Source: CAD feature listing. Evaluate the final solid. Frame: model axes, mm. A direction names the side the tool comes from. Coordinates: 2 decimals unless noted, no trailing zeros. Order: outer loops, then holes, each group sorted by start corner. A loop starts at its lowest first (then second) coordinate and runs counter-clockwise, first axis right, second up.
```python
from build123d import *

# Parameters (mm, degrees)
SKETCH1_R                     = 31.5
EXTRUDE1_DEPTH                = 4
EXTRUDE_THIN1_DEPTH           = 13
CIRPATTERN7_COUNT             = 6
SKETCH3_R                     = 7
EXTRUDE2_DEPTH                = 6
M11_0_11_DIAMETER_HOLE1_D     = 11
M11_0_11_DIAMETER_HOLE1_DEPTH = 10
M11_0_11_DIAMETER_HOLE1_TIP   = 3.304733405


with BuildPart() as part:
    # Sketch1 → Extrude1 (new body)
    with BuildSketch(Plane.XY):
        Circle(SKETCH1_R)
    extrude(amount=EXTRUDE1_DEPTH)

    # Sketch2 → Extrude-Thin1 (add)
    with BuildSketch(Plane.XY.offset(4)):
        with BuildLine():
            ThreePointArc((10, -1), (20.741698661, 1.955169442), (28.460203071, 9.988960964))
            Line((28.460203071, 9.988960964), (26.702088493, 10.942393254))
            ThreePointArc((26.702088493, 10.942393254), (19.718679741, 3.673724733), (10, 1))
            Line((10, 1), (10, -1))
        make_face()
    extrude_thin1 = extrude(amount=EXTRUDE_THIN1_DEPTH)

    # CirPattern7: Extrude-Thin1 ×6 about axis
    cirpattern7_axis = Axis((0, 0, 0), (0, 0, 1))
    for i in range(1, CIRPATTERN7_COUNT):
        add(extrude_thin1.rotate(cirpattern7_axis, i * 360 / CIRPATTERN7_COUNT))

    # Sketch3 → Extrude2 (add)
    with BuildSketch(Plane.XY.offset(4)):
        Circle(SKETCH3_R)
    extrude(amount=EXTRUDE2_DEPTH)

    # M11.0 _11_ Diameter Hole1
    with Locations(Plane.XY.offset(10)):
        with Locations((0, 0)):
            Hole(M11_0_11_DIAMETER_HOLE1_D / 2, depth=M11_0_11_DIAMETER_HOLE1_DEPTH)
            with Locations((0, 0, -(M11_0_11_DIAMETER_HOLE1_DEPTH + M11_0_11_DIAMETER_HOLE1_TIP / 2))):  # 118° drill point
                Cone(0, M11_0_11_DIAMETER_HOLE1_D / 2, M11_0_11_DIAMETER_HOLE1_TIP, mode=Mode.SUBTRACT)


solid = part.part
```
Q1. Pull-direction query (X, two-part tool) for faces 1 (the cylindrical face through (19.841, 3.747, 10.409)), 2 (the flat face through (-27.59, -10.46, 10.41)), 3 (the cylindrical face through (-4.101, 31.232, 1.972)), 4 (the flat face through (7, 0, 0)); classes: pulls with the +X half, pulls with the -X half, needs draft (parallel to the pull), parting line crosses it, or undercut.
Solutions:
face 1: undercut
face 2: pulls with the -X half
face 3: parting line crosses it
face 4: needs draft
Q2. Pin query (flat end, axial travel): P1, Ø1, axis at x = -4, z = 6, coming from the -Y side; P2, Ø1.5, axis at x = -10, z = 9, coming from the -Y side; P3, Ø2, axis at y = 0, z = 12.5, coming from the +X side; P4, Ø2, axis at x = -3, y = -18.5, coming from the -Z side. Return the tip coordinate at first contact, or that it passes through.
Solutions:
P1: stops at y = -28.98
P2: stops at y = -1.01
P3: stops at x = 18.94
P4: stops at z = 0
Q3. Section query B-B on z = 6.25. Output: boundary loops of the cut face in (x, y).
Solutions:
outline: (-28.46, -9.99) - (-26.7, -10.94) arc R19 cw to (-10, -1) - (-10, 1) arc R21 ccw to start; (-22.88, 19.65) - (-22.83, 17.65) arc R19 cw to (-5.87, 8.16) - (-4.13, 9.16) arc R21 ccw to start; circle Ø14 at (0, 0); (-5.87, -8.16) arc R21 ccw to (-5.58, -29.64) - (-3.87, -28.6) arc R19 cw to (-4.13, -9.16) - close; (3.87, 28.6) arc R19 cw to (4.13, 9.16) - (5.87, 8.16) arc R21 ccw to (5.58, 29.64) - close; (4.13, -9.16) arc R21 ccw to (22.88, -19.65) - (22.83, -17.65) arc R19 cw to (5.87, -8.16) - close; (10, -1) arc R21 ccw to (28.46, 9.99) - (26.7, 10.94) arc R19 cw to (10, 1) - close; hole circle Ø11 at (0, 0)
Q4. Section query A-A on x = 0. Output: boundary loops of the cut face in (y, z).
Solutions:
outline: (-31.5, 0) - (-5.5, 0) - (-5.5, 10) - (-7, 10) - (-7, 4) - (-31.5, 4) - close; (5.5, 0) - (31.5, 0) - (31.5, 4) - (7, 4) - (7, 10) - (5.5, 10) - close
Q5. Section query C-C on z = 11.25. Output: boundary loops of the cut face in (x, y).
Solutions:
outline: (-28.46, -9.99) - (-26.7, -10.94) arc R19 cw to (-10, -1) - (-10, 1) arc R21 ccw to start; (-22.88, 19.65) - (-22.83, 17.65) arc R19 cw to (-5.87, 8.16) - (-4.13, 9.16) arc R21 ccw to start; (-5.87, -8.16) arc R21 ccw to (-5.58, -29.64) - (-3.87, -28.6) arc R19 cw to (-4.13, -9.16) - close; (3.87, 28.6) arc R19 cw to (4.13, 9.16) - (5.87, 8.16) arc R21 ccw to (5.58, 29.64) - close; (4.13, -9.16) arc R21 ccw to (22.88, -19.65) - (22.83, -17.65) arc R19 cw to (5.87, -8.16) - close; (10, -1) arc R21 ccw to (28.46, 9.99) - (26.7, 10.94) arc R19 cw to (10, 1) - close
Q6. Section query D-D on y = 0. Output: boundary loops of the cut face in (x, z).
Solutions:
outline: (-31.5, 0) - (-5.5, 0) - (-5.5, 10) - (-7, 10) - (-7, 4) - (-10, 4) - (-10, 17) - (-16.4, 17) - (-16.4, 4) - (-31.5, 4) - close; (5.5, 0) - (31.5, 0) - (31.5, 4) - (16.4, 4) - (16.4, 17) - (10, 17) - (10, 4) - (7, 4) - (7, 10) - (5.5, 10) - close
Q7. Material intervals for line 1 along Y through (x, z) = (0, 5.25); line 2 along Z through (x, y) = (-20.5, 20); line 3 along X through (y, z) = (14.5, 12.25), sorted ascending.
Solutions:
line 1: y = -7 to -5.5, 5.5 to 7
line 2: z = 0 to 4
line 3: x = -11.83 to -8.53, 6.22 to 8.26
Q8. Set-up query: faces 5 (the cylindrical face through (11.93, -16.91, 10.41)), 6 (the cylindrical face through (6.466, -2.681, 6.958)), 7 (the flat face through (-4.7, -29.1, 10.4)), 8 (the flat face through (27.59, 10.46, 10.41)), 9 (the cylindrical face through (-20.606, -1.875, 10.409)). Return all of +Z, -Z, +X, -X, +Y, -Y with unobstructed straight access to the full face (end or side cutting, diameter ignored); none if empty.
Solutions:
face 5: +Z, -Y
face 6: +Z
face 7: +Z, +X, -Y
face 8: +Z, +X, +Y
face 9: +Z, -X
